Can you work these out from the model? Positions are in its coordinate system, mm. Face numbers are marked on the shaded views. A direction names the side the tool comes from. Round coordinates to 2 decimals unless told otherwise and drop trailing zeros. Loops run counter-clockwise (first coordinate to the right, second up) from the corner with the lowest first, then second, coordinate; pieces in that order, holes last.
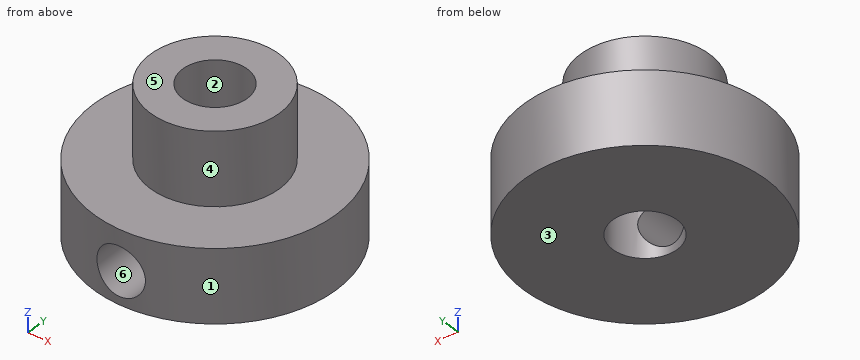
from build123d import *

# Parameters (mm, degrees)
SKETCH_1_R          = 15
EXTRUDE_1_DEPTH     = 9
SKETCH_2_R          = 8
EXTRUDE_2_DEPTH     = 9
SKETCH_3_R          = 4
CUT_EXTRUDE_1_DEPTH = 28
SKETCH_4_R          = 3
CUT_EXTRUDE_2_DEPTH = 28


with BuildPart() as part:
    # 草图1 → 凸台-拉伸1 (new body)
    with BuildSketch(Plane.XY):
        Circle(SKETCH_1_R)
    extrude(amount=EXTRUDE_1_DEPTH)

    # 草图2 → 凸台-拉伸2 (add)
    with BuildSketch(Plane.XY.offset(9)):
        Circle(SKETCH_2_R)
    extrude(amount=EXTRUDE_2_DEPTH)

    # 草图3 → 切除-拉伸1 (cut)
    with BuildSketch(Plane.XY.offset(18)):
        Circle(SKETCH_3_R)
    extrude(amount=-CUT_EXTRUDE_1_DEPTH, mode=Mode.SUBTRACT)

    # 草图4 → 切除-拉伸2 (cut)
    with BuildSketch(Plane(origin=(0, 0, 0), x_dir=(1, 0, 0), z_dir=(0, 1, 0))):
        with Locations(Location((0, -4, 0), (0, 0, 270))):
            Circle(SKETCH_4_R)
    extrude(amount=-CUT_EXTRUDE_2_DEPTH, mode=Mode.SUBTRACT)


solid = part.part
(1) If we section it at B-B, the plane y = 0: List the corners of the cut face in (x, z) for me, then the cut area to 3 significant figures.
Worked answers:
outline: (-15, 0) - (-4, 0) - (-4, 18) - (-8, 18) - (-8, 9) - (-15, 9) - close; (4, 0) - (15, 0) - (15, 9) - (8, 9) - (8, 18) - (4, 18) - close
area: 270 mm2
(2) If I drill on line 1 (Y direction, x = 0, z = 9.75); line 2 (Z direction, x = 0, y = -6.25); line 3 (Z direction, x = 0, y = -10), over which ranges is the centre line in solid material (lowest first)?
Worked answers:
line 1: y = -8 to -4, 4 to 8
line 2: z = 0 to 1, 7 to 18
line 3: z = 0 to 1, 7 to 9
(3) Will these pins go through, and if not, where does the flat tip stop? P1, Ø1, axis at x = 2.5, z = 10, coming from the +Y side; P2, Ø10, axis at y = 11.5, z = 3.5, coming from the +X side; P3, Ø4, axis at x = 7, z = 12.5, coming from the -Y side (3 decimals).
Worked answers:
P1: stops at y = 7.75
P2: stops at x = 13.52
P3: stops at y = -6.245
(4) For the marked faces 4, 5 and 6, which set-ups out of +Z, -Z, +X, -X, +Y, -Y let a thin tool reach every point of the face, with its end or its side?
Worked answers:
face 4: +Z
face 5: +Z, +X, -X, +Y, -Y
face 6: -Y
(5) If we mould it in two halves opening along X, with no side actions, what happens to the marked faces 1, 2 and 3? For each: released by +X, released by -X, zero draft, split by the parting line, or undercut.
Worked answers:
face 1: split by the parting line
face 2: undercut
face 3: zero draft
(6) If we section it at A-A, the plane x = 0: List the corners of the cut face in (y, z) for me.
Worked answers:
outline: (-15, 0) - (-4, 0) - (-4, 1) - (-15, 1) - close; (-15, 7) - (-4, 7) - (-4, 18) - (-8, 18) - (-8, 9) - (-15, 9) - close; (4, 0) - (15, 0) - (15, 9) - (8, 9) - (8, 18) - (4, 18) - close
(7) If we section it at D-D, the plane y = -4.5: List the corners of the cut face in (x, z) for me.
Worked answers:
outline: (-14.31, 0) - (14.31, 0) - (14.31, 9) - (6.61, 9) - (6.61, 18) - (-6.61, 18) - (-6.61, 9) - (-14.31, 9) - close; hole circle Ø6 at (0, 4)
(8) If we section it at C-C, the plane z = 16.75: List the corners of the cut face in (x, y) for me.
Worked answers:
outline: circle Ø16 at (0, 0); hole circle Ø8 at (0, 0)
